Read the model definition and answer for the solid it produces. Units are mm, in the model's axes. A direction names the side the tool comes from. Give positions to 0.01 mm unless a question says otherwise; leave off trailing zeros. Order: outer loops, then holes, each group sorted by start corner. A loop starts at its lowest first (then second) coordinate and runs counter-clockwise, first axis right, second up. Notation, with made-up numbers: (-8.75, 83) -> (39.25, 83) arc R15 ccw to (39.25, 90) -> close; hole circle Ø9 at (-30.5, -17.5). An arc over 180 degrees is marked (long way). Answer as CSV lines item,"result". Start each with the question number.
1) Find section A-A (x = 31.5). Determine the outline of the cut face in (y, z), and give its area (3 significant figures).
2) Straight lines are drawn through the part: L1, parallel to X at y = -9, z = 11.75; L2, parallel to Y at x = -40, z = 6.5; L3, parallel to Y at x = 32.5, z = 14.25. For each, find the intervals that lie inside material, in ascending order. Write a range as from..to.
3) Flat-ended cylindrical pins translate along their axes: pin 1 Ø5.5 at (x, y) = (23, 21) entering from +Z; pin 2 Ø5.5 at (y, z) = (-3, 2) entering from -X; pin 3 Ø23.5 at (x, y) = (19, 2.5) entering from +Z. Find the tip coordinate at first contact, or state that the pin passes through.
4) For faces 1 (the face through (-36.01, 18.236, 12.325)), 2 (the face through (-15.8, -12, 15)), 3 (the face through (31, -24, 16.11)), 4 (the face through (25.4, 0, 2)), determine the directions among +Z, -Z, +X, -X, +Y, -Y from which every point of the face is accessible in a straight line to the end or side of a thin tool.
5) Find section C-C (z = 3.25). State how many separate pieces and enclosed holes the cut face has, and give its area (3 significant figures).
6) The mould has two halves that part along Y. Classify faces 5 (the face through (-1.4, 0.8, 2.5)), 6 (the face through (0, -24, 21)): +Y half, -Y half, draft (parallel to the pull), parting line (faces both ways), or undercut.
7) Find section B-B (y = -10). Determine the outline of the cut face in (x, z).
```python
from build123d import *

# Parameters (mm, degrees)
F0_R     = 2.5
F0_R_2   = 1.524
F0_W     = 19.05
F0_H     = 38.1
F1_DEPTH = 5
F3_DEPTH = 20
F4_R     = 4
F5_DEPTH = 25.4
F6_W     = 50.8
F6_H     = 50.8
F7_DEPTH = 8.89
F8_W     = 15
F8_H     = 4.935952
F9_DEPTH = 25.4


with BuildPart() as f1:
    # F0 (on Top) → F1 (new body)
    with BuildSketch(Plane.XY):
        Polygon((50.8, 25.4), (-50.8, 25.4), (-50.8, 23.619107), (-20.8, 12.7), (-20.8, -12.7), (-50.8, -23.619107), (-50.8, -25.4), (50.8, -25.4), align=None)
        with Locations((-10.766795, 0)):
            Circle(F0_R, mode=Mode.SUBTRACT)
        with Locations((-3.766795, 0)):
            Circle(F0_R, mode=Mode.SUBTRACT)
        with Locations((22.86, -21.59)):
            Circle(F0_R_2, mode=Mode.SUBTRACT)
        with Locations((47.244, -21.59)):
            Circle(F0_R_2, mode=Mode.SUBTRACT)
        with Locations((3.233205, 0)):
            Circle(F0_R, mode=Mode.SUBTRACT)
        with Locations((10.233205, 0)):
            Circle(F0_R, mode=Mode.SUBTRACT)
        with Locations((17.233205, 0)):
            Circle(F0_R, mode=Mode.SUBTRACT)
        with Locations((34.925, 0)):
            Rectangle(F0_W, F0_H, mode=Mode.SUBTRACT)
        with Locations((22.86, 21.59)):
            Circle(F0_R_2, mode=Mode.SUBTRACT)
        with Locations((47.244, 21.59)):
            Circle(F0_R_2, mode=Mode.SUBTRACT)
    extrude(amount=F1_DEPTH)

    # F2 (on face) → F3 (join)
    with BuildSketch(Plane.XY.offset(5)):
        Polygon((50.8, -25.4), (50.8, 25.4), (-50.8, 25.4), (-50.8, 23.619107), (-20.8, 12.7), (-18.8, 12.7), (-18.8, 14.100415), (-16.8, 14.100415), (-16.8, 8.365211), (-15.8, 8.365211), (-15.8, 14.100415), (-15.8, 16.100415), (-24.294955, 16.100415), (-44.3504, 23.4), (48.8, 23.4), (48.8, -23.4), (-44.3504, -23.4), (-24.294955, -16.100415), (-15.8, -16.100415), (-15.8, -14.100415), (-15.8, -8.365211), (-16.8, -8.365211), (-16.8, -14.100415), (-18.8, -14.100415), (-18.8, -12.7), (-20.8, -12.7), (-50.8, -23.619107), (-50.8, -25.4), align=None)
    extrude(amount=F3_DEPTH)

    # F4 (on face) → F5 (cut)
    with BuildSketch(Plane.XZ.offset(-23.4)):
        with Locations((13.420951, 10.783263)):
            Circle(F4_R)
    extrude(amount=-F5_DEPTH, mode=Mode.SUBTRACT)

    # F6 (on face) → F7 (cut)
    with BuildSketch(Plane.XY.offset(25)):
        with Locations((25.4, 0)):
            Rectangle(F6_W, F6_H)
    extrude(amount=-F7_DEPTH, mode=Mode.SUBTRACT)

    # F8 (on face) → F9 (cut)
    with BuildSketch(Plane.YZ.offset(50.8)):
        with Locations((0, 13.642024)):
            Rectangle(F8_W, F8_H)
    extrude(amount=-F9_DEPTH, mode=Mode.SUBTRACT)


solid = f1.part
```
Findings below:
1,outline,"(-25.4, 0) -> (-19.05, 0) -> (-19.05, 5) -> (-23.4, 5) -> (-23.4, 16.11) -> (-25.4, 16.11) -> close; (19.05, 0) -> (25.4, 0) -> (25.4, 16.11) -> (23.4, 16.11) -> (23.4, 5) -> (19.05, 5) -> close"
1,area,"108 mm²"
2,L1,"-16.8..-15.8, 48.8..50.8"
2,L2,"-25.4..-23.4, -21.82..-19.69, 19.69..21.82, 23.4..25.4"
2,L3,"-25.4..-23.4, 23.4..25.4"
3,pin 1,"z = 16.11"
3,pin 2,"x = -20.8"
3,pin 3,"z = 5"
4,face 1,"+Z, -Z, -X"
4,face 2,"+Z"
4,face 3,"+Z, +X, +Y, -Y"
4,face 4,"+Z, -Z"
5,separate pieces,"1"
5,enclosed holes,"10"
5,area,"3,220 mm²"
6,face 5,"undercut"
6,face 6,"draft"
7,outline,"(-20.8, 0) -> (25.4, 0) -> (25.4, 5) -> (-15.8, 5) -> (-15.8, 25) -> (-16.8, 25) -> (-16.8, 5) -> (-20.8, 5) -> close; (44.45, 0) -> (50.8, 0) -> (50.8, 16.11) -> (48.8, 16.11) -> (48.8, 5) -> (44.45, 5) -> close"
